from build123d import *

# Parameters (mm, degrees)
F1_DEPTH = 6.35
F2_COUNT = 13


with BuildPart() as f1:
    # F0 (on Top) → F1 (new body)
    with BuildSketch(Plane.XY):
        with BuildLine():
            ThreePointArc((7.9296197565, 23.5951858335), (6.9911317973, 23.8900761864), (6.0417249702, 24.1476546146))
            ThreePointArc((6.0417249702, 24.1476546146), (4.3226425573, 22.4330749308), (3.2648662162, 20.2476374354))
            ThreePointArc((3.2648662162, 20.2476374354), (5.7837443287, 19.6767495961), (8.2108987358, 18.7938105523))
            ThreePointArc((8.2108987358, 18.7938105523), (8.3954934616, 19.5156536929), (8.4994507341, 20.2534379554))
            ThreePointArc((8.4994507341, 20.2534379554), (8.5176465567, 20.5391701676), (8.5237154667, 20.8254168329))
            ThreePointArc((8.5237154667, 20.8254168329), (8.373521449, 22.2418004346), (7.9296197565, 23.5951858335))
        make_face()
        with BuildLine():
            ThreePointArc((4.0264902572, 14.4598933509), (-1.7431476836, 15.057566034), (-4.9211585336, 19.9100068261))
            ThreePointArc((-4.9211585336, 19.9100068261), (-12.6431262329, -16.1486077476), (20.5091729021, 0))
            ThreePointArc((20.5091729021, 0), (19.2415803806, 7.0984334598), (15.5954927821, 13.3194135761))
            ThreePointArc((15.5954927821, 13.3194135761), (9.5256046991, 10.9946956396), (4.0264902572, 14.4598933509))
        make_face()
        with BuildLine():
            ThreePointArc((3.2648662162, 20.2476374354), (-0.8451772993, 20.4917507417), (-4.9211585336, 19.9100068261))
            ThreePointArc((-4.9211585336, 19.9100068261), (-1.7431476836, 15.057566034), (4.0264902572, 14.4598933509))
            ThreePointArc((4.0264902572, 14.4598933509), (3.0384725246, 17.2738616412), (3.2648662162, 20.2476374354))
        make_face()
        with BuildLine():
            ThreePointArc((4.0264902572, 14.4598933509), (9.5256046991, 10.9946956396), (15.5954927821, 13.3194135761))
            ThreePointArc((15.5954927821, 13.3194135761), (12.2138579016, 16.4756744411), (8.2108987358, 18.7938105523))
            ThreePointArc((8.2108987358, 18.7938105523), (6.6287005247, 16.1344397874), (4.0264902572, 14.4598933509))
        make_face()
        with BuildLine():
            ThreePointArc((8.2108987358, 18.7938105523), (5.7837443287, 19.6767495961), (3.2648662162, 20.2476374354))
            ThreePointArc((3.2648662162, 20.2476374354), (3.0384725246, 17.2738616412), (4.0264902572, 14.4598933509))
            ThreePointArc((4.0264902572, 14.4598933509), (6.6287005247, 16.1344397874), (8.2108987358, 18.7938105523))
        make_face()
    extrude(amount=F1_DEPTH)

    # F2: F1 ×13 about axis
    f2_axis = Axis((0, 0, 6.35), (0, 0, 1))


with BuildPart() as f1_1:
    add(f1.part)
    for i in range(1, F2_COUNT):
        add(f1.part.rotate(f2_axis, i * 360 / F2_COUNT))


solid = f1_1.part
Input: part model. Units: mm. Frame: model coordinates. A direction names the side the tool comes from. Coordinates: 2 decimals unless noted, no trailing zeros. Loops run counter-clockwise (first coordinate to the right, second up) from the corner with the lowest first, then second, coordinate; pieces in that order, holes last. Notation, with made-up numbers: (70.5, 48) - (83.5, 48) arc R17 cw to (83.5, 66) - close; hole circle Ø2 at (15, -21). An arc over 180 degrees is marked (long way). Answer in a Markdown table with one row per item. Add a question column.
Item 1: Mould query, pull axis X, two halves, no side actions, for faces 1 (the cylindrical face through (14.28, 17.87, 3.13)), 2 (the cylindrical face through (23.64, 7.8, 3.13)), 3 (the cylindrical face through (-15.679, 19.333, 3.131)). Classes: released by +X, released by -X, zero draft, split by the parting line, or undercut.
Item 2: Contact query for flat-ended pins moving along their axis: P1, Ø3, axis at y = -17, z = 2, coming from the -X side; P2, Ø1, axis at x = 11, z = 4.5, coming from the +Y side. Output: stop coordinate, or through.
Item 3: Access query for faces 4 (the flat face through (0, 0, 6.35)), 5 (the cylindrical face through (19.461, -12.025, 3.131)), 6 (the cylindrical face through (-20.225, 3.403, 3.131)). Directions: +Z, -Z, +X, -X, +Y, -Y. A direction counts if a zero-diameter tool reaches every point of the face in a straight line with its end or side. Return the directions, or none.
Item 4: Section query B-B on x = -5. Return the cut outline in (y, z).
Item 5: Section query A-A on y = -8. Return the cut outline in (x, z).
Item 6: Line query: line 1 along Y through (x, z) = (-21, 5); line 2 along X through (y, z) = (-15, 5.75); line 3 along X through (y, z) = (-13.5, 5.75). Output: solid intervals per line, ascending. Write a range as [from, to].
Recorded:
| question | item | result |
|---|---|---|
| 1 | face 1 | undercut |
| 1 | face 2 | released by +X |
| 1 | face 3 | released by -X |
| 2 | P1 | x = -13.43 |
| 2 | P2 | y = 17.62 |
| 3 | face 4 | +Z, +X, -X, +Y, -Y |
| 3 | face 5 | +Z, -Z, +X |
| 3 | face 6 | +Z, -Z, -X |
| 4 | outline | (-19.89, 0) - (24.38, 0) - (24.38, 6.35) - (-19.89, 6.35) - close |
| 5 | outline | (-18.88, 0) - (18.88, 0) - (18.88, 6.35) - (-18.88, 6.35) - close |
| 6 | line 1 | [-13.36, -11.07], [-4.14, 0.96], [6.4, 11] |
| 6 | line 2 | [-13.99, 13.99], [15.67, 19.86] |
| 6 | line 3 | [-20.91, -16.83], [-15.44, 20.21] |
